Here's the drawing with two shaded views (mm, measured from the low corner). I have some questions. A direction names the side the tool comes from. Coordinates: 2 decimals unless noted, no trailing zeros. Write each loop counter-clockwise with the first axis right and the second up, starting at its lowest first coordinate (ties: lowest second). Pieces come first, ordered by that corner, then holes. Notation, with made-up numbers: (35.5, -6.5) -> (40.5, -6.5) arc R18 cw to (40.5, 10.5) -> close; hole circle Ø4 at (-10, 87.25). An arc over 180 degrees is marked (long way). Put each result on its own line as item: value.
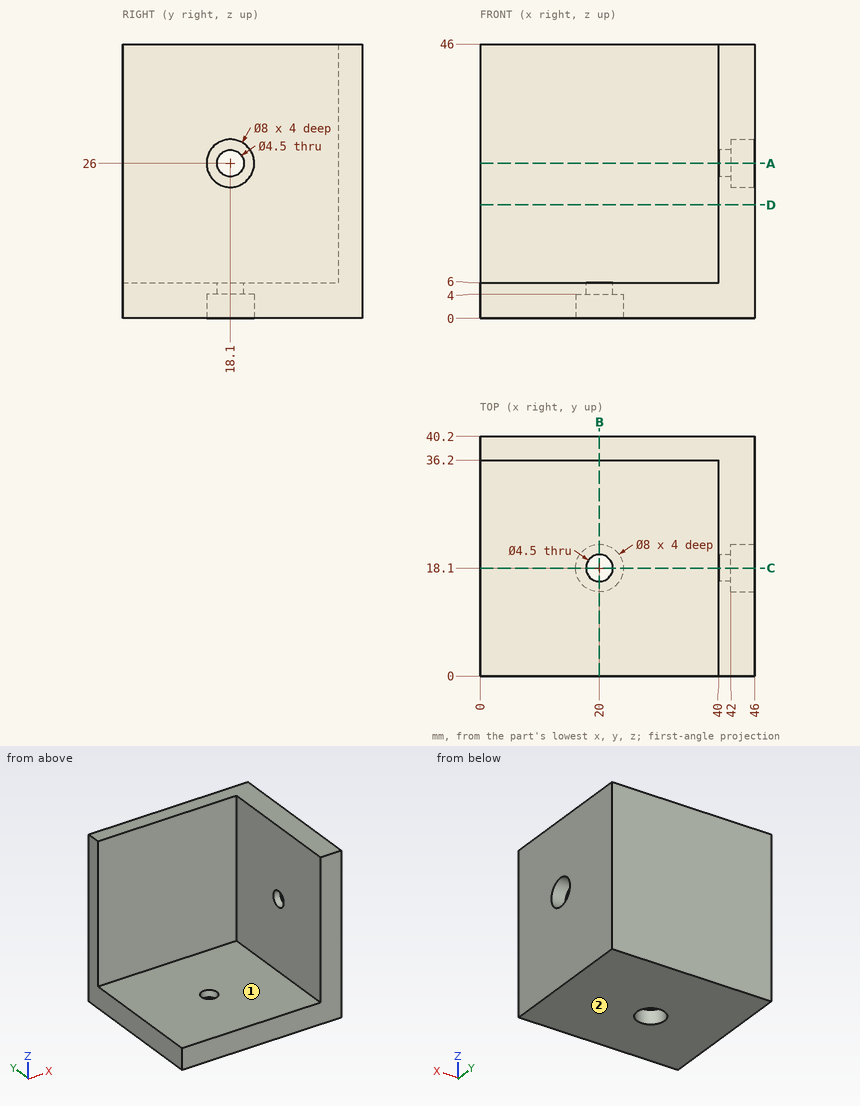
Item 1: For P1, Ø6.5, axis at x = 20, y = 18.1, coming from the -Z side; P2, Ø4, axis at y = 19.5, z = 34, coming from the -X side; P3, Ø5, axis at y = 18.1, z = 26, coming from the +X side, each with a flat end and sliding along its axis, tell me the tip position at first contact or that it passes through.
Output:
P1: stops at z = 4
P2: stops at x = 40
P3: stops at x = 42
Item 2: Imagine slicing it at A-A on z = 26. Write out the boundary of the cut face in (x, y), then the cut area to 3 significant figures.
Output:
outline: (0, 36.2) -> (40, 36.2) -> (40, 20.35) -> (42, 20.35) -> (42, 22.1) -> (46, 22.1) -> (46, 40.2) -> (0, 40.2) -> close; (40, 0) -> (46, 0) -> (46, 14.1) -> (42, 14.1) -> (42, 15.85) -> (40, 15.85) -> close
area: 360 mm²
Item 3: Imagine slicing it at C-C on y = 18.1. Write out the boundary of the cut face in (x, z).
Output:
outline: (0, 0) -> (16, 0) -> (16, 4) -> (17.75, 4) -> (17.75, 6) -> (0, 6) -> close; (22.25, 4) -> (24, 4) -> (24, 0) -> (46, 0) -> (46, 22) -> (42, 22) -> (42, 23.75) -> (40, 23.75) -> (40, 6) -> (22.25, 6) -> close; (40, 28.25) -> (42, 28.25) -> (42, 30) -> (46, 30) -> (46, 46) -> (40, 46) -> close
Item 4: Imagine slicing it at D-D on z = 19. Write out the boundary of the cut face in (x, y), then the cut area to 3 significant figures.
Output:
outline: (0, 36.2) -> (40, 36.2) -> (40, 0) -> (46, 0) -> (46, 40.2) -> (0, 40.2) -> close
area: 401 mm²
Item 5: Please list where these lines run through material, in increasing order: line 1 along Z through (x, y) = (43.15, 18.1); line 2 along Y through (x, z) = (20, 5.4); line 3 along Y through (x, z) = (25.5, 14). Write a range as from..to.
Output:
line 1: z = 0..22, 30..46
line 2: y = 0..15.85, 20.35..40.2
line 3: y = 36.2..40.2
Item 6: Which directions (+Z, -Z, +X, -X, +Y, -Y) give clear straight access to the entire face, cutting with the end or side of a thin tool? Please do the marked faces 1 and 2.
Output:
face 1: +Z, -X, -Y
face 2: -Z, +X, -X, +Y, -Y
Item 7: Imagine slicing it at B-B on x = 20. Write out the boundary of the cut face in (y, z).
Output:
outline: (0, 0) -> (14.1, 0) -> (14.1, 4) -> (15.85, 4) -> (15.85, 6) -> (0, 6) -> close; (20.35, 4) -> (22.1, 4) -> (22.1, 0) -> (40.2, 0) -> (40.2, 46) -> (36.2, 46) -> (36.2, 6) -> (20.35, 6) -> close
